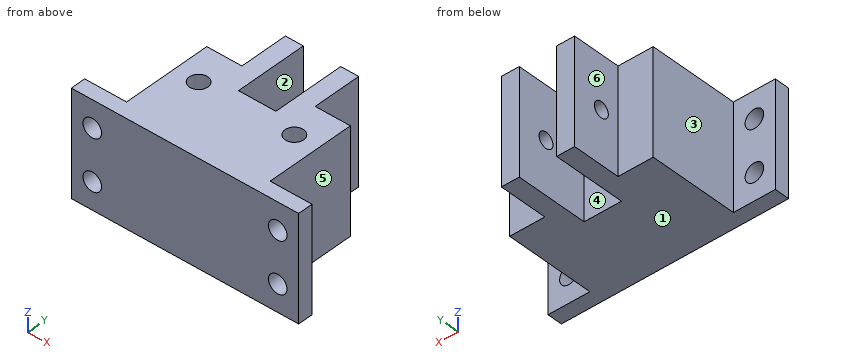
from build123d import *

# Parameters (mm, degrees)
SKETCH1_R           = 3.1
BOSS_EXTRUDE1_DEPTH = 35
SKETCH2_R           = 3.1
BOSS_EXTRUDE2_DEPTH = 5
BOSS_EXTRUDE3_DEPTH = 35
SKETCH4_R           = 2.6
CUT_EXTRUDE1_DEPTH  = 37.25
SKETCH6_W           = 12.5
SKETCH6_H           = 8
CUT_EXTRUDE2_DEPTH  = 36
SKETCH7_W           = 48
SKETCH7_H           = 35
BOSS_EXTRUDE4_DEPTH = 10
SKETCH8_W           = 14
SKETCH8_H           = 35
SKETCH8_R           = 3.1
BOSS_EXTRUDE5_DEPTH = 5


with BuildPart() as part:
    # Sketch1 → Boss-Extrude1 (new body)
    with BuildSketch(Plane.XY):
        Polygon((-5, -3.75), (-35, -3.75), (-35, -28.75), (13, -28.75), (13, -3.75), align=None)
        with Locations((5, -15.75)):
            Circle(SKETCH1_R, mode=Mode.SUBTRACT)
        with Locations((-27, -15.75)):
            Circle(SKETCH1_R, mode=Mode.SUBTRACT)
    extrude(amount=BOSS_EXTRUDE1_DEPTH)

    # Sketch2 → Boss-Extrude2 (add)
    with BuildSketch(Plane(origin=(0, 0, 0), x_dir=(-1, 0, 0), z_dir=(0, 0, -1))):
        with Locations((27, -15.75)):
            Circle(SKETCH2_R)
        with Locations((-5, -15.75)):
            Circle(SKETCH2_R)
    extrude(amount=-BOSS_EXTRUDE2_DEPTH)

    # Sketch3 → Boss-Extrude3 (add)
    with BuildSketch(Plane.XY.offset(35)):
        Polygon((-17.25, 2.5), (-17.25, -7.5), (-23.25, -7.5), (-23.25, 12.5), (-17.25, 12.5), align=None)
        Polygon((-4.75, 2.5), (-4.75, -7.5), (1.25, -7.5), (1.25, 12.5), (-4.75, 12.5), align=None)
    extrude(amount=-BOSS_EXTRUDE3_DEPTH)

    # Sketch4 → Cut-Extrude1 (cut, through all)
    with BuildSketch(Plane.ZY.offset(23.25)):
        with Locations((17.5, 2.5)):
            Circle(SKETCH4_R)
    extrude(amount=-CUT_EXTRUDE1_DEPTH, mode=Mode.SUBTRACT)

    # Sketch6 → Cut-Extrude2 (cut, through all)
    with BuildSketch(Plane.XY.offset(35)):
        with Locations((-11, -7.75)):
            Rectangle(SKETCH6_W, SKETCH6_H)
    extrude(amount=-CUT_EXTRUDE2_DEPTH, mode=Mode.SUBTRACT)

    # Sketch7 → Boss-Extrude4 (add)
    with BuildSketch(Plane.XZ.offset(28.75)):
        with Locations((-11, 17.5)):
            Rectangle(SKETCH7_W, SKETCH7_H)
    extrude(amount=BOSS_EXTRUDE4_DEPTH)

    # Sketch8 → Boss-Extrude5 (add)
    with BuildSketch(Plane.XZ.offset(38.75)):
        with Locations((-42, 17.5)):
            Rectangle(SKETCH8_W, SKETCH8_H)
        with Locations((-42, 9)):
            Circle(SKETCH8_R, mode=Mode.SUBTRACT)
        with Locations((-42, 26)):
            Circle(SKETCH8_R, mode=Mode.SUBTRACT)
        with Locations((20, 17.5)):
            Rectangle(SKETCH8_W, SKETCH8_H)
        with Locations((20, 9)):
            Circle(SKETCH8_R, mode=Mode.SUBTRACT)
        with Locations((20, 26)):
            Circle(SKETCH8_R, mode=Mode.SUBTRACT)
    extrude(amount=-BOSS_EXTRUDE5_DEPTH)


solid = part.part
CAD build for the part. Positions are in the model's coordinates, mm. Face numbers are marked on the shaded views. A direction names the side the tool comes from. Round coordinates to 2 decimals unless told otherwise and drop trailing zeros. Loops run counter-clockwise (first coordinate to the right, second up) from the corner with the lowest first, then second, coordinate; pieces in that order, holes last.
(1) Cut at B-B (x = -42). Give the cut face in (y, z).
(2) Drop flat-ended pins along their axis: pin 1 (5.5 mm diameter, centred on x = -42, z = 9, fed in from +Y); pin 2 (10 mm diameter, centred on x = -42, z = 26, fed in from +Y); pin 3 (7.5 mm diameter, centred on y = -1.5, z = 25.5, fed in from -X); pin 4 (13 mm diameter, centred on x = 9.5, z = 24.5, fed in from +Y). Give the stop position or say it passes through.
(3) Cut at D-D (z = 13). Give the cut face in (x, y), plus the area to 3 significant figures.
(4) Cut at C-C (y = 9.5). Give the cut face in (x, z), plus the area to 3 significant figures.
(5) Two-plate mould, pull along X, no slides. Class the marked faces 1, 2 and 3: +X half, -X half, draft (parallel to the pull), parting line (faces both ways), or undercut.
(6) Cut at A-A (z = 17.5). Give the cut face in (x, y), plus the area to 3 significant figures.
(7) Wall check: line 1 along Z through (x, y) = (20, -35); line 2 along X through (y, z) = (-13.5, 20); line 3 along Y through (x, z) = (-27, 28). Give the ranges that are in metal, low to high.
(8) Which spindle directions (+Z, -Z, +X, -X, +Y, -Y) get a long thin tool onto all of the face, cutting with end or side? Do the marked faces 4, 5 and 6. Say none if no direction does.
Findings below:
1. outline: (-38.75, 0) - (-33.75, 0) - (-33.75, 5.9) - (-38.75, 5.9) - close; (-38.75, 12.1) - (-33.75, 12.1) - (-33.75, 22.9) - (-38.75, 22.9) - close; (-38.75, 29.1) - (-33.75, 29.1) - (-33.75, 35) - (-38.75, 35) - close
2. pin 1: passes through
2. pin 2: stops at y = -33.75
2. pin 3: stops at x = -35
2. pin 4: stops at y = -3.75
3. outline: (-49, -38.75) - (27, -38.75) - (27, -33.75) - (13, -33.75) - (13, -3.75) - (1.25, -3.75) - (1.25, 12.5) - (-4.75, 12.5) - (-4.75, -11.75) - (-17.25, -11.75) - (-17.25, 12.5) - (-23.25, 12.5) - (-23.25, -3.75) - (-35, -3.75) - (-35, -33.75) - (-49, -33.75) - close; hole circle Ø6.2 at (-27, -15.75); hole circle Ø6.2 at (5, -15.75)
3. area: 1,850 mm2
4. outline: (-23.25, 0) - (-17.25, 0) - (-17.25, 35) - (-23.25, 35) - close; (-4.75, 0) - (1.25, 0) - (1.25, 35) - (-4.75, 35) - close
4. area: 420 mm2
5. face 1: draft
5. face 2: undercut
5. face 3: -X half
6. outline: (-49, -38.75) - (27, -38.75) - (27, -33.75) - (13, -33.75) - (13, -3.75) - (1.25, -3.75) - (1.25, -0.1) - (-4.75, -0.1) - (-4.75, -11.75) - (-17.25, -11.75) - (-17.25, -0.1) - (-23.25, -0.1) - (-23.25, -3.75) - (-35, -3.75) - (-35, -33.75) - (-49, -33.75) - close; (-23.25, 5.1) - (-17.25, 5.1) - (-17.25, 12.5) - (-23.25, 12.5) - close; (-4.75, 5.1) - (1.25, 5.1) - (1.25, 12.5) - (-4.75, 12.5) - close; hole circle Ø6.2 at (-27, -15.75); hole circle Ø6.2 at (5, -15.75)
6. area: 1,790 mm2
7. line 1: z = 0 to 5.9, 12.1 to 22.9, 29.1 to 35
7. line 2: x = -35 to -29.13, -24.87 to 2.87, 7.13 to 13
7. line 3: y = -38.75 to -18.85, -12.65 to -3.75
8. face 4: +Z, -Z, +Y
8. face 5: +Z, -Z, +X, +Y
8. face 6: +Z, -Z, -X, +Y
